```python
from build123d import *

# Parameters (mm, degrees)
F1_DEPTH  = 3
F2_DEPTH  = 40
F5_DEPTH  = 37
F7_DEPTH  = 3
F8_DEPTH  = 3
F9_DEPTH  = 90
F10_DEPTH = 8
F11_R     = 4
F11_R_2   = 1.4
F12_DEPTH = 15
F13_DEPTH = 18
F14_W     = 10.0909090909
F14_H     = 18
F15_DEPTH = 101.4
F16_DEPTH = 5


with BuildPart() as f1:
    # F0 (on Front) → F1 (new body)
    with BuildSketch(Plane.XZ):
        Polygon((32.5, 17.5), (-32.5, 17.5), (-32.5, -14.5), (-24.45, -14.5), (-24.45, 15), (-20.75, 15), (-17.05, 15), (-17.05, -14.5), (-11, -14.5), (-11, 15), (11, 15), (11, -14.5), (17.05, -14.5), (17.05, 15), (20.75, 15), (24.45, 15), (24.45, -14.5), (32.5, -14.5), align=None)
    extrude(amount=F1_DEPTH)

    # F0 (on Front) → F2 (join)
    with BuildSketch(Plane.XZ):
        Polygon((-24.45, -14.5), (-32.5, -14.5), (-32.5, -17.5), (32.5, -17.5), (32.5, -14.5), (24.45, -14.5), (24.45, -15), (20.75, -15), (17.05, -15), (17.05, -14.5), (11, -14.5), (11, -15), (-11, -15), (-11, -14.5), (-17.05, -14.5), (-17.05, -15), (-20.75, -15), (-24.45, -15), align=None)
    extrude(amount=F2_DEPTH)

    # F4 (on face) → F5 (join)
    with BuildSketch(Plane.XZ.offset(3)):
        Polygon((-14, -14.5), (-11, -14.5), (-11, 15), (-11, 17.5), (-14, 17.5), align=None)
        Polygon((11, 17.5), (11, 15), (11, -14.5), (14, -14.5), (14, 17.5), align=None)
    extrude(amount=F5_DEPTH)

    # F6 (on face) → F7 (join)
    with BuildSketch(Plane.YZ.offset(32.5)):
        Polygon((-3, -14.5), (-3, 17.5), (-40, -14.5), align=None)
    extrude(amount=-F7_DEPTH)

    # F3 (on face) → F8 (join)
    with BuildSketch(Plane(origin=(-32.5, 0, 0), x_dir=(0, -1, 0), z_dir=(-1, 0, 0))):
        Polygon((40, -14.5), (3, 17.5), (3, -14.5), align=None)
    extrude(amount=-F8_DEPTH)

    # F3 (on face) → F9 (cut)
    with BuildSketch(Plane(origin=(-32.5, 0, 0), x_dir=(0, -1, 0), z_dir=(-1, 0, 0))):
        Polygon((45.3402064741, 20.7598140836), (3, 17.5), (40, -14.5), align=None)
    extrude(amount=-F9_DEPTH, mode=Mode.SUBTRACT)

    # F10 (add): a face of the model
    f10_faces = [f1.faces().sort_by_distance(p)[0] for p in [
        (0, -20, -17.5),
    ]]
    extrude(f10_faces, amount=F10_DEPTH)

    # F11 (on face) → F12 (cut)
    with BuildSketch(Plane(origin=(0, 0, -25.5), x_dir=(1, 0, 0), z_dir=(0, 0, -1))):
        with Locations((-21.75, -16.4545454545)):
            Circle(F11_R)
        with Locations((-21.75, -16.4545454545)):
            Circle(F11_R_2, mode=Mode.SUBTRACT)
        with Locations((21.75, -16.4545454545)):
            Circle(F11_R)
        with Locations((21.75, -16.4545454545)):
            Circle(F11_R_2, mode=Mode.SUBTRACT)
    extrude(amount=-F12_DEPTH, mode=Mode.SUBTRACT)

    # F11 (on face) → F13 (cut)
    with BuildSketch(Plane(origin=(0, 0, -25.5), x_dir=(1, 0, 0), z_dir=(0, 0, -1))):
        with Locations((-21.75, -16.4545454545)):
            Circle(F11_R_2)
        with Locations((21.75, -16.4545454545)):
            Circle(F11_R_2)
    extrude(amount=-F13_DEPTH, mode=Mode.SUBTRACT)

    # F14 (on face) → F15 (cut)
    with BuildSketch(Plane.YZ.offset(32.5)):
        with Locations((-34.9545454545, -20)):
            Rectangle(F14_W, F14_H)
    extrude(amount=-F15_DEPTH, mode=Mode.SUBTRACT)

    # F16 (add): a face of the model
    f16_faces = [f1.faces().sort_by_distance(p)[0] for p in [
        (0, -1.5, 17.5),
    ]]
    extrude(f16_faces, amount=-F16_DEPTH)


solid = f1.part
```
Input: part model. Units: mm. Frame: model coordinates. A direction names the side the tool comes from. Give positions to 0.01 mm unless a question says otherwise; leave off trailing zeros. Loops run counter-clockwise (first coordinate to the right, second up) from the corner with the lowest first, then second, coordinate; pieces in that order, holes last. Notation, with made-up numbers: (1, 31) -> (19, 31) arc R22 cw to (19, 40) -> close; hole circle Ø1 at (46.5, 12.5). An arc over 180 degrees is marked (long way). Use a Markdown table: item, result.
Q1. Access query for faces 1 (the flat face through (-25, -3, 2)), 2 (the flat face through (0, -29.909, -20)), 3 (the flat face through (31.021, -19.246, 3.449)), 4 (the flat face through (-24.45, -2.7, -4.4)). Directions: +Z, -Z, +X, -X, +Y, -Y. A direction counts if a zero-diameter tool reaches every point of the face in a straight line with its end or side. Return the directions, or none.
Entries:
| item | result |
|---|---|
| face 1 | +Z, -Y |
| face 2 | -Z, +X, -X, -Y |
| face 3 | +Z, +X, -X, -Y |
| face 4 | +Y, -Y |
Q2. Pull-direction query (Z, two-part tool) for faces 5 (the flat face through (0, -1, 12.5)), 6 (the flat face through (11, -14, -2)), 7 (the flat face through (-14, -12, -2)), 8 (the flat face through (13, -33, -11)); classes: pulls with the +Z half, pulls with the -Z half, needs draft (parallel to the pull), parting line crosses it, or undercut.
Entries:
| item | result |
|---|---|
| face 5 | undercut |
| face 6 | undercut |
| face 7 | needs draft |
| face 8 | pulls with the -Z half |
Q3. Section query A-A, the plane x = -9.5. Return the cut outline in (y, z), plus the area to 3 significant figures.
Entries:
| item | result |
|---|---|
| outline | (-29.91, -25.5) -> (0, -25.5) -> (0, -15) -> (-29.91, -15) -> close; (-3, 12.5) -> (0, 12.5) -> (0, 17.5) -> (-3, 17.5) -> close |
| area | 329 mm² |
Q4. Section query C-C, the plane y = -33.5. Return the cut outline in (x, z).
Entries:
| item | result |
|---|---|
| outline | (-32.5, -11) -> (-29.5, -11) -> (-29.5, -8.88) -> (-32.5, -8.88) -> close; (-14, -11) -> (-11, -11) -> (-11, -8.88) -> (-14, -8.88) -> close; (11, -11) -> (14, -11) -> (14, -8.88) -> (11, -8.88) -> close; (29.5, -11) -> (32.5, -11) -> (32.5, -8.88) -> (29.5, -8.88) -> close |
Q5. First-contact query: P1, Ø1.5, axis at x = 12.5, y = -31.5, coming from the -Z side; P2, Ø8, axis at y = -21, z = 5, coming from the +X side; P3, Ø3, axis at x = -25, y = -27.5, coming from the +Z side; P4, Ø3, axis at x = 13.5, z = 12.5, coming from the -Y side. Flat tips, straight axial feed; report the tip coordinate or a pass-through.
Entries:
| item | result |
|---|---|
| P1 | stops at z = -11 |
| P2 | stops at x = 32.5 |
| P3 | stops at z = -14.5 |
| P4 | stops at y = -10.52 |
Q6. Ray query, probe 1 along X at (y, z) = (-11.5, -13.5); probe 2 along Z at (x, y) = (-9.5, -2); probe 3 along Y at (x, z) = (-19, -23). Return the intervals inside material, ascending. Write a range as from..to.
Entries:
| item | result |
|---|---|
| probe 1 | x = -32.5..-29.5, -14..-11, 11..14, 29.5..32.5 |
| probe 2 | z = -25.5..-15, 12.5..17.5 |
| probe 3 | y = -29.91..0 |
Q7. Section query D-D, the plane z = 14.5. Return the cut outline in (x, y), plus the area to 3 significant figures.
Entries:
| item | result |
|---|---|
| outline | (-32.5, -6.47) -> (-29.5, -6.47) -> (-29.5, -3) -> (-14, -3) -> (-14, -6.47) -> (-11, -6.47) -> (-11, -3) -> (11, -3) -> (11, -6.47) -> (14, -6.47) -> (14, -3) -> (29.5, -3) -> (29.5, -6.47) -> (32.5, -6.47) -> (32.5, 0) -> (-32.5, 0) -> close |
| area | 237 mm² |
Q8. Section query B-B, the plane z = 1. Return the cut outline in (x, y), plus the area to 3 significant figures.
Entries:
| item | result |
|---|---|
| outline | (-32.5, -22.08) -> (-29.5, -22.08) -> (-29.5, -3) -> (-24.45, -3) -> (-24.45, 0) -> (-32.5, 0) -> close; (-17.05, -3) -> (-14, -3) -> (-14, -22.08) -> (-11, -22.08) -> (-11, 0) -> (-17.05, 0) -> close; (11, -22.08) -> (14, -22.08) -> (14, -3) -> (17.05, -3) -> (17.05, 0) -> (11, 0) -> close; (24.45, -3) -> (29.5, -3) -> (29.5, -22.08) -> (32.5, -22.08) -> (32.5, 0) -> (24.45, 0) -> close |
| area | 314 mm² |
